Autodesk Inventor part; units mm, degrees
ref_plane "YZ Plane" through (0, 0, 0) normal (1, 0, 0) x (0, 1, 0)
ref_plane "XZ Plane" through (0, 0, 0) normal (0, 1, 0) x (-1, 0, 0)
ref_plane "XY Plane" through (0, 0, 0) normal (0, 0, 1) x (1, 0, 0)
sketch "Sketch1" plane through (0, 0, 0) normal (0, 0, 1) x (1, 0, 0)
  line L0 (0, 0) -> (-80, 0)
  line L1 (-80, 0) -> (-80, 80)
  line L2 (-80, 80) -> (0, 80)
  line L3 (0, 80) -> (0, 0)
  line L4 (-75, 75) -> (-5, 75)
  line L5 (-5, 75) -> (-5, 5)
  line L6 (-5, 5) -> (-75, 5)
  line L7 (-75, 5) -> (-75, 75)
  dimension "d0" = 80
  dimension "d1" = 80
  dimension "d2" = 70
  dimension "d3" = 70
extrude "Extrusion1" add sketch "Sketch1" along normal blind 10 contours L0 L1 L2 L3 | L4 L5 L6 L7
sketch "Sketch2" plane through (-80, 80, 0) normal (0, 1, 0) x (1, 0, 0)
  line L0 (24.4, -3.45) -> (15.6, -3.45)
  line L1 (15.6, -3.45) -> (15.6, -6.55)
  line L2 (15.6, -6.55) -> (24.4, -6.55)
  line L3 (24.4, -6.55) -> (24.4, -3.45)
  line L4 (64.4, -3.45) -> (55.6, -3.45)
  line L5 (55.6, -3.45) -> (55.6, -6.55)
  line L6 (55.6, -6.55) -> (64.4, -6.55)
  line L7 (64.4, -6.55) -> (64.4, -3.45)
  point P0 (80, 0)
  point P1 (20, -5)
  point P2 (60, -5)
  dimension "d8" = 8.8
  dimension "d9" = 3.1
  dimension "d12" = 8.8
  dimension "d13" = 3.1
extrude "Extrusion2" cut sketch "Sketch2" against normal blind 10
sketch "Sketch4" plane through (0, 0, 10) normal (0, 0, 1) x (1, 0, 0)
  line L0 (-5, 5) -> (-75, 5)
  line L1 (-75, 5) -> (-75, 75)
  line L2 (-75, 75) -> (-5, 75)
  line L3 (-5, 75) -> (-5, 5)
  point P0 (0, 0)
  dimension "d21" = 70
  dimension "d22" = 70
extrude "Extrusion3" cut sketch "Sketch4" against normal blind 2
sketch "Sketch5" plane through (-80, 0, 0) normal (0, -1, 0) x (1, 0, 0)
  line L0 (2, 2) -> (12, 2)
  line L1 (12, 2) -> (12, 5)
  line L2 (12, 5) -> (2, 5)
  line L3 (2, 5) -> (2, 2)
  line L4 (78, 2) -> (68, 2)
  line L5 (68, 2) -> (68, 5)
  line L6 (68, 5) -> (78, 5)
  line L7 (78, 5) -> (78, 2)
  point P0 (80, 0)
  dimension "d25" = 10
  dimension "d26" = 3
  dimension "d27" = 10
  dimension "d28" = 3
extrude "Extrusion4" cut sketch "Sketch5" against normal blind 10
properties part number "Marker_TestFit"
The model under review builds one solid part; all positions refer to its coordinate system, in mm. A direction names the side the tool comes from. Round coordinates to 2 decimals unless told otherwise and drop trailing zeros. Write each loop counter-clockwise with the first axis right and the second up, starting at its lowest first coordinate (ties: lowest second). Pieces come first, ordered by that corner, then holes. Notation, with made-up numbers: (2.5, -31) - (46.5, -31) arc R34 cw to (46.5, 5) - close; hole circle Ø5 at (-4, 7.5). An arc over 180 degrees is marked (long way). Use one line per item in the form item = value.
Q1. Consider section C-C (x = -39). State the section outline as (y, z) points.
Answer key:
outline = (0, 0) - (80, 0) - (80, 10) - (75, 10) - (75, 8) - (5, 8) - (5, 10) - (0, 10) - close
Q2. Consider section B-B (z = 9). State the section outline as (x, y) points, and give its area (3 significant figures).
Answer key:
outline = (-80, 0) - (0, 0) - (0, 80) - (-80, 80) - close; hole (-75, 5) - (-5, 5) - (-5, 75) - (-75, 75) - close
area = 1,500 mm2
Q3. For line 1 (X direction, y = 17.5, z = 8.5); line 2 (Y direction, x = -16, z = 8.75); line 3 (Z direction, x = -19.5, y = 77), list the stretches that pass through material, from the lowest coordinate up. Write a range as [from, to].
Answer key:
line_1 = [-80, -75], [-5, 0]
line_2 = [0, 5], [75, 80]
line_3 = [0, 3.45], [6.55, 10]
Q4. Consider section A-A (y = 73). State the section outline as (x, z) points, and give its area (3 significant figures).
Answer key:
outline = (-80, 0) - (0, 0) - (0, 10) - (-5, 10) - (-5, 8) - (-75, 8) - (-75, 10) - (-80, 10) - close; hole (-64.4, 3.45) - (-55.6, 3.45) - (-55.6, 6.55) - (-64.4, 6.55) - close; hole (-24.4, 3.45) - (-15.6, 3.45) - (-15.6, 6.55) - (-24.4, 6.55) - close
area = 605 mm2
Q5. Draft analysis for pull direction X (two halves, no side actions). For faces 6 (the flat face through (-76, 40, 10)), 7 (the flat face through (-7, 10, 4)), state which applies: +X half, -X half, draft (parallel to the pull), parting line (faces both ways), or undercut.
Answer key:
face_6 = draft
face_7 = undercut
Q6. Tool access review of faces 1 (the flat face through (-20, 75, 3.45)), 2 (the flat face through (-41, 80, 5)), 3 (the flat face through (-40, 40, 8)), 4 (the flat face through (-73, 10, 4)), 5 (the flat face through (-39, 0, 5)): name each direction out of +Z, -Z, +X, -X, +Y, -Y from which nothing blocks a thin tool from reaching the whole face with its end or side.
Answer key:
face_1 = +Y
face_2 = +Z, -Z, +X, -X, +Y
face_3 = +Z
face_4 = -Y
face_5 = +Z, -Z, +X, -X, -Y
Q7. Insertion check: pin 1 Ø4 at (x, y) = (-54, 17) entering from +Z. The pin has a flat end and moves straight along its axis. Give the tip position at first contact, or say it passes through.
Answer key:
pin_1 = 8
Q8. Consider section D-D (y = 61). State the section outline as (x, z) points.
Answer key:
outline = (-80, 0) - (0, 0) - (0, 10) - (-5, 10) - (-5, 8) - (-75, 8) - (-75, 10) - (-80, 10) - close
